Part model, mm, in its own coordinate system. A direction names the side the tool comes from. Round coordinates to 2 decimals unless told otherwise and drop trailing zeros. Write each loop counter-clockwise with the first axis right and the second up, starting at its lowest first coordinate (ties: lowest second). Pieces come first, ordered by that corner, then holes. Notation, with made-up numbers: (-31.75, 37) -> (1.25, 37) arc R27 cw to (1.25, 56) -> close; hole circle Ø6 at (-36, 46.5). An arc over 180 degrees is marked (long way). Return JSON: item names as keys, results as strings. Group by question number.
```python
from build123d import *

# Parameters (mm, degrees)
CHAMFER_1_SIZE               = 0.5
HOLE_WIZARD_M6_1_D           = 6
HOLE_WIZARD_M6_1_DEPTH       = 15
HOLE_WIZARD_M6_1_CSINK_D     = 7
HOLE_WIZARD_M6_1_CSINK_ANGLE = 90
HOLE_WIZARD_M6_1_TIP         = 1.802581857
CUT_EXTRUDE_START            = 4.5
CUT_EXTRUDE_1_DEPTH          = 10
CUT_EXTRUDE_START_2          = 5
CUT_EXTRUDE_2_DEPTH          = 10
PATTERN_CIRCULAR_1_COUNT     = 2


with BuildPart() as part:
    # 草图1 → 旋转1 (revolve)
    with BuildSketch(Plane.XY, mode=Mode.PRIVATE) as revolve_1_sk:
        Polygon((0, 0), (0, 7), (15, 7), (15, 10), (18, 10), (18, 8.5), (69, 8.5), (69, 0), align=None)
    revolve(revolve_1_sk.sketch.rotate(Axis((0, 0, 0), (1, 0, 0)), 90), axis=Axis((0, 0, 0), (1, 0, 0)))

    # 倒角1
    chamfer_1_edges = [part.edges().sort_by_distance(p)[0] for p in [
        (69, 0, -8.5),
        (18, 0, -10),
        (15, 0, -10),
        (0, 0, -7),
    ]]
    chamfer(chamfer_1_edges, length=CHAMFER_1_SIZE)

    # M6 螺纹孔的螺纹孔钻头1
    with Locations(Plane(origin=(69, 0, 0), x_dir=(0, 0, -1), z_dir=(1, 0, 0))):
        with Locations((0, 0)):
            CounterSinkHole(HOLE_WIZARD_M6_1_D / 2, HOLE_WIZARD_M6_1_CSINK_D / 2, depth=HOLE_WIZARD_M6_1_DEPTH, counter_sink_angle=HOLE_WIZARD_M6_1_CSINK_ANGLE)
            with Locations((0, 0, -(HOLE_WIZARD_M6_1_DEPTH + HOLE_WIZARD_M6_1_TIP / 2))):  # 118° drill point
                Cone(0, HOLE_WIZARD_M6_1_D / 2, HOLE_WIZARD_M6_1_TIP, mode=Mode.SUBTRACT)

    # 草图4 → 切除-拉伸1 (cut)
    with BuildSketch(Plane.XY.offset(CUT_EXTRUDE_START)):
        with BuildLine():
            Line((0, 2.5), (12.5, 2.5))
            ThreePointArc((12.5, 2.5), (15, 0), (12.5, -2.5))
            Line((12.5, -2.5), (0, -2.5))
            Line((0, -2.5), (0, 2.5))
        make_face()
    extrude(amount=CUT_EXTRUDE_1_DEPTH, mode=Mode.SUBTRACT)

    # 草图5 → 切除-拉伸2 (cut)
    with BuildSketch(Plane.XY.offset(CUT_EXTRUDE_START_2)):
        with BuildLine():
            Line((69, 2.5), (56.5, 2.5))
            ThreePointArc((56.5, 2.5), (54, 0), (56.5, -2.5))
            Line((56.5, -2.5), (69, -2.5))
            Line((69, -2.5), (69, 2.5))
        make_face()
    cut_extrude_2 = extrude(amount=CUT_EXTRUDE_2_DEPTH, mode=Mode.SUBTRACT)

    # 阵列(圆周)1: 切除-拉伸2 ×2 about axis
    pattern_circular_1_axis = Axis((0, 0, 0), (1, 0, 0))
    for i in range(1, PATTERN_CIRCULAR_1_COUNT):
        add(cut_extrude_2.rotate(pattern_circular_1_axis, i * 360 / PATTERN_CIRCULAR_1_COUNT), mode=Mode.SUBTRACT)


solid = part.part
```
Item 1: Wall check: L1, parallel to Y at x = 63.5, z = 0; L2, parallel to Z at x = 61, y = 0; L3, parallel to X at y = -5.25, z = 6. Give the ranges that are in metal, low to high.
Item 2: Flat gauge pins, fed straight in: P1, Ø2.5, axis at x = 59, y = -1, coming from the -Z side; P2, Ø2, axis at x = 5.5, z = 6, coming from the +Y side; P3, Ø1.6, axis at x = 64.5, z = 6.5, coming from the -Y side. Where does each tip first touch, or does it go through?
Item 3: Which spindle directions (+Z, -Z, +X, -X, +Y, -Y) get a long thin tool onto all of the face, cutting with end or side? Do faces 1 (the face through (8, 0, -7)), 2 (the face through (63, -2.5, -7)), 3 (the face through (6, 2.5, 6)), 4 (the face through (63, 2.5, 7)). Say none if no direction does.
Item 4: Cut at A-A (x = 25). Write the cut outline in (y, z), then the cut area to 3 significant figures.
Checks:
{
 "1": {"L1": "y = -8.5 to -3, 3 to 8.5", "L2": "z = -5 to -3, 3 to 5", "L3": "x = 15 to 69"},
 "2": {"P1": "stops at z = -5", "P2": "stops at y = 4.9", "P3": "stops at y = -6.31"},
 "3": {"face 1": "-X", "face 2": "-Z, +X", "face 3": "+Z, -X", "face 4": "+Z, +X"},
 "4": {"outline": "circle Ø17 at (0, 0)", "area": "227 mm2"}
}
